Drawing for the job (mm, zero at the part's lowest x, y, z). A direction names the side the tool comes from. Round coordinates to 2 decimals unless told otherwise and drop trailing zeros. Loops run counter-clockwise (first coordinate to the right, second up) from the corner with the lowest first, then second, coordinate; pieces in that order, holes last. Notation, with made-up numbers: M 80,-4 L 125,-4 A8 cw 125,7 Z; hole C -40,-36.75 d9. An arc over 180 degrees is marked long. Answer in a Markdown table with one row per item.
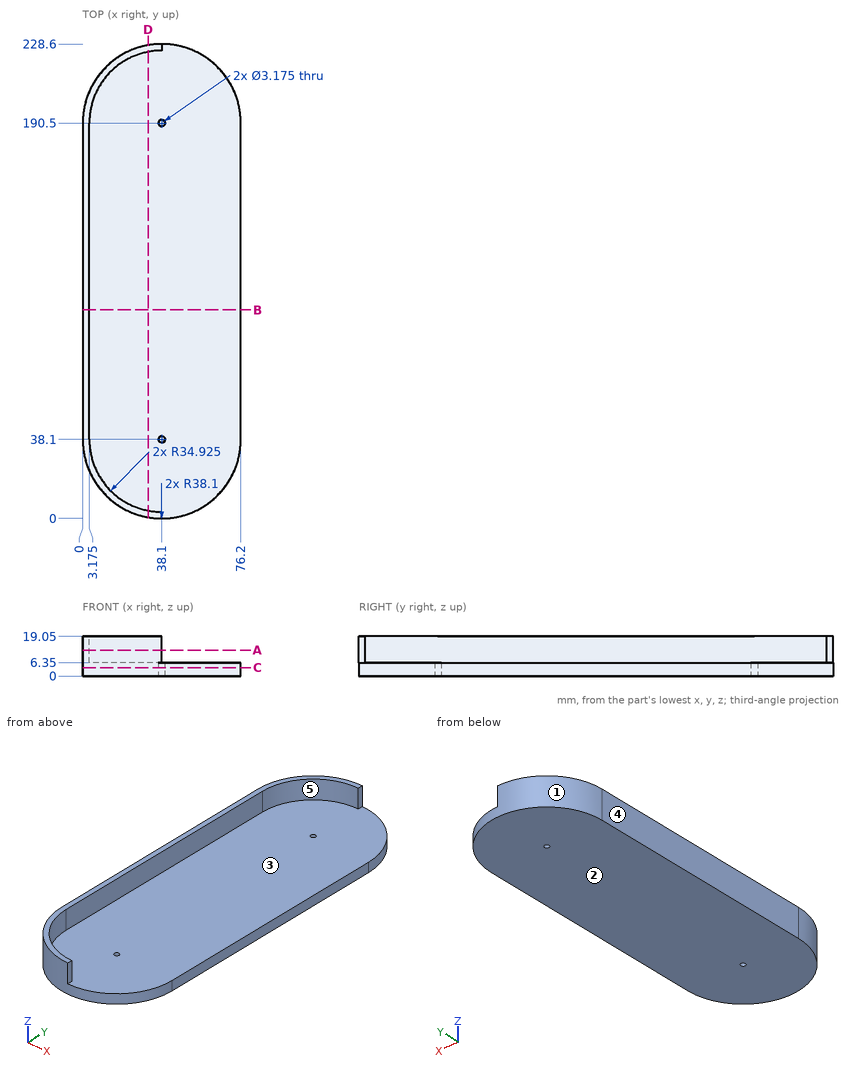
1. Saw through at B-B (y = 100.5). Write the cut outline in (x, z) (3 decimals).
Verdict:
| item | result |
|---|---|
| outline | M 0,0 L 76.2,0 L 76.2,6.35 L 3.175,6.35 L 3.175,19.05 L 0,19.05 Z |
2. Wall check: probe 1 along Y at (x, z) = (38.1, 3); probe 2 along X at (y, z) = (38.1, 2.25); probe 3 along Z at (x, y) = (69, 95). Give the ranges that are in metal, low to high.
Verdict:
| item | result |
|---|---|
| probe 1 | y = 0 to 36.51, 39.69 to 188.91, 192.09 to 228.6 |
| probe 2 | x = 0 to 36.51, 39.69 to 76.2 |
| probe 3 | z = 0 to 6.35 |
3. Saw through at C-C (z = 4). Write the cut outline in (x, y) (1 decimal), and give its area (3 significant figures).
Verdict:
| item | result |
|---|---|
| outline | M 0,38.1 A38.1 ccw 76.2,38.1 L 76.2,190.5 A38.1 ccw 0,190.5 Z; hole C 38.1,38.1 d3.2; hole C 38.1,190.5 d3.2 |
| area | 16,200 mm² |
4. Tool access for the marked faces 4 and 5: list every direction of +Z, -Z, +X, -X, +Y, -Y with a clear straight run to the whole face (end or side of a thin tool).
Verdict:
| item | result |
|---|---|
| face 4 | +Z, -Z, -X, +Y, -Y |
| face 5 | +Z, +X |
5. Saw through at D-D (x = 31.5). Write the cut outline in (y, z).
Verdict:
| item | result |
|---|---|
| outline | M 0.58,0 L 228.02,0 L 228.02,19.05 L 224.8,19.05 L 224.8,6.35 L 3.8,6.35 L 3.8,19.05 L 0.58,19.05 Z |
6. Mould opens along Y. For the marked faces 1, 2 and 3 say: +Y half, -Y half, draft (parallel to the pull), parting line (faces both ways), or undercut.
Verdict:
| item | result |
|---|---|
| face 1 | +Y half |
| face 2 | draft |
| face 3 | undercut |
7. Pin check, flat tips, straight feed: pin 1 (8 mm diameter, centred on x = 15, y = 179.5, fed in from +Z); pin 2 (2 mm diameter, centred on y = 170.5, z = 14.5, fed in from +X) (3 decimals); pin 3 (1.5 mm diameter, centred on x = 8, z = 4.5, fed in from +Y). Stop position of each tip, or through.
Verdict:
| item | result |
|---|---|
| pin 1 | stops at z = 6.35 |
| pin 2 | stops at x = 3.175 |
| pin 3 | stops at y = 214.79 |
8. Saw through at A-A (z = 12.5). Write the cut outline in (x, y) (3 decimals), and give its area (3 significant figures).
Verdict:
| item | result |
|---|---|
| outline | M 0,38.1 A38.1 ccw 38.1,0 L 38.1,3.175 A34.925 cw 3.175,38.1 L 3.175,190.5 A34.925 cw 38.1,225.425 L 38.1,228.6 A38.1 ccw 0,190.5 Z |
| area | 848 mm² |
